Autodesk Inventor part; units mm, degrees
ref_plane "rail_to_adjusting_block_XY" through (0, 0, -220) normal (0, 1, 0) x (1, 0, 0)
ref_plane "rail_to_adjusting_block_YZ" through (0, 0, -220) normal (1, 0, 0) x (0, 0, -1)
ref_plane "rail_to_adjusting_block_ZX" through (0, 0, -220) normal (0, 0, -1) x (0, 1, 0)
sketch "Sketch_12" plane through (0, 0, 0) normal (0, 0, 1) x (1, 0, 0)
  line L0 (-4.5, 5.3) -> (-4.5, 5.0434)
  line L1 (-4.5, 5.0434) -> (-4.2216, 4.8827)
  arc A0 (-3.7548, 4.35) -> (-4.2216, 4.8827) centre (-4.7715, 3.93) ccw
  line L2 (-3.7548, 4.35) -> (-3.1, 4.35)
  line L3 (-3.1, 4.35) -> (-3.1, 3.65)
  line L4 (-3.1, 3.65) -> (-3.7548, 3.65)
  arc A1 (-4.2216, 3.1173) -> (-3.7548, 3.65) centre (-4.7715, 4.07) ccw
  line L5 (-4.2216, 3.1173) -> (-4.5, 2.9566)
  line L6 (-4.5, 2.9566) -> (-4.5, 0.3)
  line L7 (-4.5, 0.3) -> (-4.2, 0)
  line L8 (-4.2, 0) -> (4.2, 0)
  line L9 (4.2, 0) -> (4.5, 0.3)
  line L10 (4.5, 0.3) -> (4.5, 2.9566)
  line L11 (4.5, 2.9566) -> (4.2216, 3.1173)
  arc A2 (3.7548, 3.65) -> (4.2216, 3.1173) centre (4.7715, 4.07) ccw
  line L12 (3.7548, 3.65) -> (3.1, 3.65)
  line L13 (3.1, 3.65) -> (3.1, 4.35)
  line L14 (3.1, 4.35) -> (3.7548, 4.35)
  arc A3 (4.2216, 4.8827) -> (3.7548, 4.35) centre (4.7715, 3.93) ccw
  line L15 (4.2216, 4.8827) -> (4.5, 5.0434)
  line L16 (4.5, 5.0434) -> (4.5, 5.3)
  line L17 (4.5, 5.3) -> (4.3, 5.5)
  line L18 (4.3, 5.5) -> (-4.3, 5.5)
  line L19 (-4.3, 5.5) -> (-4.5, 5.3)
extrude "Extrusion1" add sketch "Sketch_12" along normal mid plane 60
sketch "Sketch2" plane through (-4.3, 5.5, 30) normal (0, 1, 0) x (1, 0, 0)
  point P0 (4.3, 447.5)
hole "Hole1" at (0, 5.5, -417.5) direction (0, -1, 0) diameter 3.5 depth 5.5 counterbore diameter 6 counterbore depth 3.5
pattern_linear "Rectangular Pattern1" count 23 spacing 20 along (0, 0, 1) of "Hole1"
ref_plane "rail_to_adjusting_block_XY" through (0, 0, -220) normal (0, 1, 0) x (1, 0, 0)
ref_plane "rail_to_adjusting_block_YZ" through (0, 0, -220) normal (1, 0, 0) x (0, 0, -1)
ref_plane "rail_to_adjusting_block_ZX" through (0, 0, -220) normal (0, 0, -1) x (0, 1, 0)
ref_plane "to_block_XY" through (0, 5.5, 113.75) normal (0, 0, 1) x (1, 0, 0)
ref_plane "to_block_YZ" through (0, 5.5, 113.75) normal (1, 0, 0) x (0, 1, 0)
ref_plane "to_block_ZX" through (0, 5.5, 113.75) normal (0, 1, 0) x (0, 0, 1)
ref_plane "to_block_2_XY" through (0, 5.5, -113.75) normal (0, 0, 1) x (1, 0, 0)
ref_plane "to_block_2_YZ" through (0, 5.5, -113.75) normal (1, 0, 0) x (0, 1, 0)
ref_plane "to_block_2_ZX" through (0, 5.5, -113.75) normal (0, 1, 0) x (0, 0, 1)
ref_plane "to_kue_XY" through (0, 0, 0) normal (0, 1, 0) x (1, 0, 0)
ref_plane "to_kue_YZ" through (0, 0, 0) normal (1, 0, 0) x (0, 0, -1)
ref_plane "to_kue_ZX" through (0, 0, 0) normal (0, 0, -1) x (0, 1, 0)
properties part number "SSE2B-MX10-455_r" material "ステンレス鋼"
For this review, take the finished solid that the model builds, in its own axes (mm). A direction names the side the tool comes from. Give positions to 0.01 mm unless a question says otherwise; leave off trailing zeros. Write each loop counter-clockwise with the first axis right and the second up, starting at its lowest first coordinate (ties: lowest second). Pieces come first, ordered by that corner, then holes.
Item 1: Machinability: for faces 4 (the face through (-0.1, 3.7, -20.5)), 5 (the face through (-2, 5.5, 0)), which of the approach directions +Z, -Z, +X, -X, +Y, -Y give a long, thin tool a straight path to every point of the face, cutting with its end or side? Answer none if there is none.
Item 2: Take a section at B-B (y = 1.3). Give the boundary of the cut face in (x, z), and give its area (3 significant figures).
Item 3: Wall thickness on probe 1 along Z at (x, y) = (0, 4.75); probe 2 along Z at (x, y) = (1, 1.2); probe 3 along X at (y, z) = (0.5, 2.5): over which ranges is each line inside the solid? List them lowest first.
Item 4: Take a section at A-A (x = 0). Give the boundary of the cut face in (y, z), and give its area (3 significant figures).
Item 5: Insertion check: P1, Ø0.5, axis at x = 3.5, z = -3.5, coming from the -Y side; P2, Ø0.6, axis at y = 4, z = -2.5, coming from the +X side; P3, Ø3, axis at x = 1, z = -17, coming from the +Y side. Each pin has a flat end and moves straight along its axis. Give the tip position at first contact, or say it passes through.
Item 6: The part is to be moulded in two halves that separate along Z. For faces 1 (the face through (0, 3, 30)), 2 (the face through (-0.08, 0.99, 20.75)), 3 (the face through (-4.5, 2, 0)), say which applies: +Z half, -Z half, draft (parallel to the pull), parting line (faces both ways), or undercut.
Item 7: Take a section at D-D (z = -24.5). Give the boundary of the cut face in (x, y).
Established:
1. face 4: +Y
1. face 5: +Z, -Z, +X, -X, +Y
2. outline: (-4.5, -30) - (4.5, -30) - (4.5, 30) - (-4.5, 30) - close; hole circle Ø3.5 at (0, -17.5); hole circle Ø3.5 at (0, 2.5); hole circle Ø3.5 at (0, 22.5)
2. area: 511 mm2
3. probe 1: z = -30 to -20.5, -14.5 to -0.5, 5.5 to 19.5, 25.5 to 30
3. probe 2: z = -30 to -18.94, -16.06 to 1.06, 3.94 to 21.06, 23.94 to 30
3. probe 3: x = -4.5 to -1.75, 1.75 to 4.5
4. outline: (0, -30) - (5.5, -30) - (5.5, -20.5) - (2, -20.5) - (2, -19.25) - (0, -19.25) - close; (0, -15.75) - (2, -15.75) - (2, -14.5) - (5.5, -14.5) - (5.5, -0.5) - (2, -0.5) - (2, 0.75) - (0, 0.75) - close; (0, 4.25) - (2, 4.25) - (2, 5.5) - (5.5, 5.5) - (5.5, 19.5) - (2, 19.5) - (2, 20.75) - (0, 20.75) - close; (0, 24.25) - (2, 24.25) - (2, 25.5) - (5.5, 25.5) - (5.5, 30) - (0, 30) - close
4. area: 246 mm2
5. P1: stops at y = 0
5. P2: stops at x = 3.1
5. P3: stops at y = 2
6. face 1: +Z half
6. face 2: undercut
6. face 3: draft
7. outline: (-4.5, 0.3) - (-4.2, 0) - (4.2, 0) - (4.5, 0.3) - (4.5, 2.96) - (4.22, 3.12) arc R1.1 cw to (3.75, 3.65) - (3.1, 3.65) - (3.1, 4.35) - (3.75, 4.35) arc R1.1 cw to (4.22, 4.88) - (4.5, 5.04) - (4.5, 5.3) - (4.3, 5.5) - (-4.3, 5.5) - (-4.5, 5.3) - (-4.5, 5.04) - (-4.22, 4.88) arc R1.1 cw to (-3.75, 4.35) - (-3.1, 4.35) - (-3.1, 3.65) - (-3.75, 3.65) arc R1.1 cw to (-4.22, 3.12) - (-4.5, 2.96) - close
